The model under review builds one solid part; all positions refer to its coordinate system, in mm. A direction names the side the tool comes from. Give positions to 0.01 mm unless a question says otherwise; leave off trailing zeros. Order: outer loops, then holes, each group sorted by start corner. A loop starts at its lowest first (then second) coordinate and runs counter-clockwise, first axis right, second up. Notation, with made-up numbers: (27, -12.5) - (77, -12.5) arc R18 ccw to (77, 3.5) - close; hole circle Ø10 at (42.5, 79). An arc over 180 degrees is marked (long way). Put each result on its own line as item: value.
```python
from build123d import *

# Parameters (mm, degrees)
F0_W      = 65
F0_H      = 110
F1_DEPTH  = 40
F2_SIZE2  = 60
F2_SIZE   = 50
F3_R      = 10
F3_R_2    = 7.5
F4_DEPTH  = 65
F5_W      = 50
F5_H      = 50
F6_DEPTH  = 80
F7_DEPTH  = 5
F8_W      = 65
F8_H      = 65
F8_W_2    = 50
F8_H_2    = 50
F9_DEPTH  = 5
F11_DEPTH = 12.5


with BuildPart() as f1:
    # F0 (on Right) → F1 (new body, symmetric)
    with BuildSketch(Plane.YZ):
        Rectangle(F0_W, F0_H)
    extrude(amount=F1_DEPTH, both=True)

    # F2
    f2_edges = [f1.edges().sort_by_distance(p)[0] for p in [
        (40, 0, -55),
    ]]
    f2_side = f1.faces().sort_by_distance((40, 0, 0))[0]
    chamfer(f2_edges, length=F2_SIZE, length2=F2_SIZE2, reference=f2_side)

    # F3 (on face) → F4 (cut, through all)
    with BuildSketch(Plane.XZ.offset(32.5)):
        with Locations((-20, 35)):
            Circle(F3_R)
        with Locations((20, 35)):
            Circle(F3_R)
        with Locations((-20, -25)):
            Circle(F3_R_2)
    extrude(amount=-F4_DEPTH, mode=Mode.SUBTRACT)

    # F5 (on face) → F6 (cut, through all)
    with BuildSketch(Plane.YZ.offset(40)):
        with Locations((0, 25)):
            Rectangle(F5_W, F5_H)
    extrude(amount=-F6_DEPTH, mode=Mode.SUBTRACT)

    # F7 (add): a face of the model
    f7_faces = [f1.faces().sort_by_distance(p)[0] for p in [
        (-40, 0, -13.4408602151),
    ]]
    extrude(f7_faces, amount=F7_DEPTH)

    # F8 (on face) → F9 (cut)
    with BuildSketch(Plane(origin=(-45, 0, 0), x_dir=(0, -1, 0), z_dir=(-1, 0, 0))):
        with Locations((0, 22.5)):
            Rectangle(F8_W, F8_H)
        with Locations((0, 25)):
            Rectangle(F8_W_2, F8_H_2, mode=Mode.SUBTRACT)
    extrude(amount=-F9_DEPTH, mode=Mode.SUBTRACT)

    # F10 (on Front) → F11 (cut, symmetric)
    with BuildSketch(Plane.XZ):
        Polygon((-32.5196777628, -12.5074763466), (-32.5196777628, -24.9999955257), (-32.5196777628, -37.5074763466), (33.280384575, -37.5074763466), (33.280384575, -12.5074763466), align=None)
    extrude(amount=F11_DEPTH, both=True, mode=Mode.SUBTRACT)


solid = f1.part
```
(1) The part is to be moulded in two halves that separate along Z. For faces 4 (the flat face through (-11, -32.5, 11)), 5 (the flat face through (-43, 0, -10)), 6 (the flat face through (1, -25, 25)), 7 (the flat face through (10, -15, -30)), say which applies: pulls with the +Z half, pulls with the -Z half, needs draft (parallel to the pull), parting line crosses it, or undercut.
The answers:
face 4: needs draft
face 5: pulls with the +Z half
face 6: undercut
face 7: pulls with the -Z half
(2) Take a section at A-A, the plane y = -17. Write out the cut boundary in (x, z).
The answers:
outline: (-45, -55) - (-20, -55) - (40, -5) - (40, 0) - (-40, 0) - (-40, -10) - (-45, -10) - close; (-40, 50) - (40, 50) - (40, 55) - (-40, 55) - close; hole circle Ø15 at (-20, -25)
(3) Take a section at B-B, the plane z = 35. Write out the cut boundary in (x, y), then the cut area to 3 significant figures.
The answers:
outline: (-40, -32.5) - (-30, -32.5) - (-30, -25) - (-40, -25) - close; (-40, 25) - (-30, 25) - (-30, 32.5) - (-40, 32.5) - close; (-10, -32.5) - (10, -32.5) - (10, -25) - (-10, -25) - close; (-10, 25) - (10, 25) - (10, 32.5) - (-10, 32.5) - close; (30, -32.5) - (40, -32.5) - (40, -25) - (30, -25) - close; (30, 25) - (40, 25) - (40, 32.5) - (30, 32.5) - close
area: 600 mm^2
(4) Take a section at C-C, the plane x = -3.5. Write out the cut boundary in (y, z), then the cut area to 3 significant figures.
The answers:
outline: (-32.5, -41.25) - (32.5, -41.25) - (32.5, 55) - (-32.5, 55) - close; hole (-25, 0) - (25, 0) - (25, 50) - (-25, 50) - close; hole (-12.5, -37.51) - (12.5, -37.51) - (12.5, -12.51) - (-12.5, -12.51) - close
area: 3,130 mm^2
(5) For faces 1 (the flat face through (0, 0, -12.507)), 2 (the cylindrical face through (24.614, 28.697, 26.128)), 3 (the flat face through (1, 25, 25)), list the 3-axis set-ups (+Z, -Z, +X, -X, +Y, -Y) from which the entire face can be reached by the end or side of a thin tool; tool diameter is ignored.
The answers:
face 1: +X
face 2: +Y, -Y
face 3: +X, -X
(6) Take a section at D-D, the plane z = 17.5. Write out the cut boundary in (x, y).
The answers:
outline: (-40, -32.5) - (40, -32.5) - (40, -25) - (-40, -25) - close; (-40, 25) - (40, 25) - (40, 32.5) - (-40, 32.5) - close
(7) Clearance check with flat-ended pins moving along their axes: pin 1 Ø12.5 at (y, z) = (3.5, -26.5) entering from +X; pin 2 Ø1.5 at (x, y) = (-42.5, -6) entering from +Z; pin 3 Ø12.5 at (x, y) = (-3.5, -3.5) entering from -Z; pin 4 Ø17 at (x, z) = (-20, -25) entering from -Y. State where each tip first meets the part, or that it passes through.
The answers:
pin 1: x = -32.52
pin 2: z = -10
pin 3: z = -46.46
pin 4: y = -32.5
(8) Wall thickness on L1, parallel to Z at x = -20, y = -17.5; L2, parallel to Z at x = -38, y = 2; L3, parallel to Y at x = -24.5, z = -16.5: over which ranges is each line inside the solid? List them lowest first.
The answers:
L1: -55 to -32.5, -17.5 to 0, 50 to 55
L2: -55 to 0, 50 to 55
L3: -32.5 to -12.5, 12.5 to 32.5
